```python
from build123d import *

# Parameters (mm, degrees)
SKETCH1_R           = 25
SKETCH1_R_2         = 5.5
SKETCH1_R_3         = 1.55
BOSS_EXTRUDE1_DEPTH = 4
SKETCH2_R           = 2.8
CUT_EXTRUDE1_DEPTH  = 2.8
SKETCH4_R           = 18
SKETCH4_R_2         = 13.5
BOSS_EXTRUDE2_DEPTH = 20
SKETCH5_R           = 25
SKETCH5_R_2         = 18
BOSS_EXTRUDE3_DEPTH = 8
SKETCH3_R           = 2.5
CUT_EXTRUDE3_DEPTH  = 8


with BuildPart() as part:
    # Sketch1 → Boss-Extrude1 (new body)
    with BuildSketch(Plane.XY):
        Circle(SKETCH1_R)
        Circle(SKETCH1_R_2, mode=Mode.SUBTRACT)
        with Locations((0, 11)):
            Circle(SKETCH1_R_3, mode=Mode.SUBTRACT)
        with Locations((9.526279442, 5.5)):
            Circle(SKETCH1_R_3, mode=Mode.SUBTRACT)
        with Locations((9.526279442, -5.5)):
            Circle(SKETCH1_R_3, mode=Mode.SUBTRACT)
        with Locations((0, -11)):
            Circle(SKETCH1_R_3, mode=Mode.SUBTRACT)
        with Locations((-9.526279442, -5.5)):
            Circle(SKETCH1_R_3, mode=Mode.SUBTRACT)
        with Locations((-9.526279442, 5.5)):
            Circle(SKETCH1_R_3, mode=Mode.SUBTRACT)
    extrude(amount=BOSS_EXTRUDE1_DEPTH)

    # Sketch2 → Cut-Extrude1 (cut)
    with BuildSketch(Plane(origin=(0, 0, 0), x_dir=(-1, 0, 0), z_dir=(0, 0, -1))):
        with Locations((0, 11)):
            Circle(SKETCH2_R)
        with Locations((9.526279442, 5.5)):
            Circle(SKETCH2_R)
        with Locations((9.526279442, -5.5)):
            Circle(SKETCH2_R)
        with Locations((0, -11)):
            Circle(SKETCH2_R)
        with Locations((-9.526279442, -5.5)):
            Circle(SKETCH2_R)
        with Locations((-9.526279442, 5.5)):
            Circle(SKETCH2_R)
    extrude(amount=-CUT_EXTRUDE1_DEPTH, mode=Mode.SUBTRACT)

    # Sketch4 → Boss-Extrude2 (add)
    with BuildSketch(Plane.XY.offset(4)):
        Circle(SKETCH4_R)
        Circle(SKETCH4_R_2, mode=Mode.SUBTRACT)
    extrude(amount=BOSS_EXTRUDE2_DEPTH)

    # Sketch5 → Boss-Extrude3 (add)
    with BuildSketch(Plane.XY.offset(4)):
        Circle(SKETCH5_R)
        Circle(SKETCH5_R_2, mode=Mode.SUBTRACT)
    extrude(amount=BOSS_EXTRUDE3_DEPTH)

    # Sketch3 → Cut-Extrude3 (cut)
    with BuildSketch(Plane(origin=(0, 0, 0), x_dir=(-1, 0, 0), z_dir=(0, 0, -1))):
        with Locations((0, 18)):
            Circle(SKETCH3_R)
        with Locations((18, 0)):
            Circle(SKETCH3_R)
        with Locations((0, -18)):
            Circle(SKETCH3_R)
        with Locations((-18, 0)):
            Circle(SKETCH3_R)
    extrude(amount=-CUT_EXTRUDE3_DEPTH, mode=Mode.SUBTRACT)


solid = part.part
```
The listing builds one solid part. Answer for the finished solid, in the listing's coordinates (mm). A direction names the side the tool comes from. Coordinates: 2 decimals unless noted, no trailing zeros. Loops run counter-clockwise (first coordinate to the right, second up) from the corner with the lowest first, then second, coordinate; pieces in that order, holes last. Notation, with made-up numbers: (68.5, 65) -> (78.5, 65) arc R19 ccw to (78.5, 95) -> close; hole circle Ø5 at (42, 62). An arc over 180 degrees is marked (long way). Return JSON: item names as keys, results as strings. Group by question number.
(1) A cutting plane is placed at A-A on y = 0. Write down the section's boundary in (x, z), and give its area (3 significant figures).
(2) A cutting plane is placed at C-C on x = 0. Count the separate pieces of the cut face and the enclosed holes in it, and give its area (3 significant figures).
(3) A cutting plane is placed at B-B on z = 8.75. Write down the section's boundary in (x, y), and give its area (3 significant figures).
(4) Determine the mould class of faces 1 (the cylindrical face through (23.846, 7.509, 5.916)), 2 (the flat face through (2.58, 13.42, 24)), 3 (the flat face through (8, -7, 2.8)) for opening direction Y: released by +Y, released by -Y, zero draft, split by the parting line, or undercut.
(5) Which of the six approach directions +Z, -Z, +X, -X, +Y, -Y give full straight-line access (tool end or side, diameter ignored) to faces 4 (the flat face through (-18, 0, 8)), 5 (the cylindrical face through (-11.075, -5.432, 3.392)), 6 (the flat face through (11, -16, 12))?
(6) Find the intervals of material crossed by probe 1 along Y at (x, z) = (0, 6.25); probe 2 along Y at (x, z) = (0, 3.3); probe 3 along Z at (x, y) = (-8.5, -8.5), in increasing order. Write a range as from..to.
(7) A cutting plane is placed at D-D on y = 16.5. Write down the section's boundary in (x, z).
(8) Given pin 1 Ø4.5 at (x, y) = (0, -11) entering from +Z; pin 2 Ø12 at (x, z) = (14.5, 9) entering from +Y; pin 3 Ø9 at (x, y) = (0, 0) entering from +Z; pin 4 Ø4.5 at (x, y) = (-9.53, 5.5) entering from -Z, each flat-ended and moving along its own axis, determine where each tip first touches the part or whether it passes through.
The answers:
{
 "1": {"outline": "(-25, 0) -> (-20.5, 0) -> (-20.5, 8) -> (-15.5, 8) -> (-15.5, 0) -> (-5.5, 0) -> (-5.5, 4) -> (-13.5, 4) -> (-13.5, 24) -> (-18, 24) -> (-18, 12) -> (-25, 12) -> close; (5.5, 0) -> (15.5, 0) -> (15.5, 8) -> (20.5, 8) -> (20.5, 0) -> (25, 0) -> (25, 12) -> (18, 12) -> (18, 24) -> (13.5, 24) -> (13.5, 4) -> (5.5, 4) -> close", "area": "368 mm^2"},
 "2": {"separate pieces": "4", "enclosed holes": "0", "area": "329 mm^2"},
 "3": {"outline": "circle Ø50 at (0, 0); hole circle Ø27 at (0, 0)", "area": "1,390 mm^2"},
 "4": {"face 1": "split by the parting line", "face 2": "zero draft", "face 3": "undercut"},
 "5": {"face 4": "-Z", "face 5": "+Z, -Z", "face 6": "+Z"},
 "6": {"probe 1": "y = -25..-20.5, -15.5..-13.5, 13.5..15.5, 20.5..25", "probe 2": "y = -25..-20.5, -15.5..-12.55, -9.45..-5.5, 5.5..9.45, 12.55..15.5, 20.5..25", "probe 3": "z = 0..4"},
 "7": {"outline": "(-18.78, 0) -> (-2, 0) -> (-2, 8) -> (2, 8) -> (2, 0) -> (18.78, 0) -> (18.78, 12) -> (7.19, 12) -> (7.19, 24) -> (-7.19, 24) -> (-7.19, 12) -> (-18.78, 12) -> close"},
 "8": {"pin 1": "stops at z = 4", "pin 2": "stops at y = 23.51", "pin 3": "passes through", "pin 4": "stops at z = 2.8"}
}
